The listing builds one solid part. Answer for the finished solid, in the listing's coordinates (mm). A direction names the side the tool comes from. Round coordinates to 2 decimals unless told otherwise and drop trailing zeros. Write each loop counter-clockwise with the first axis right and the second up, starting at its lowest first coordinate (ties: lowest second). Pieces come first, ordered by that corner, then holes. Notation, with made-up numbers: (25.25, -31) - (37.25, -31) arc R23 cw to (37.25, 2) - close; hole circle Ø6 at (19, 42.25). An arc over 180 degrees is marked (long way). Use a Markdown table: item, result. Add a question column.
1) Find the intervals of material crossed by probe 1 along X at (y, z) = (0.25, 1.25); probe 2 along Y at (x, z) = (0, 2.7) (3 decimals); probe 3 along X at (y, z) = (-0.25, 3.5), in increasing order. Write a range as from..to.
2) A tool of negligible diameter and unlimited length cuts with its end or side. For faces 4 (the flat face through (6, -6, -1.2)), 5 (the flat face through (57, 0, 7)), 6 (the cylindrical face through (-1.751, -7.883, 2.465)), from which of +Z, -Z, +X, -X, +Y, -Y can it reach the whole face along a straight path? Write none if from no direction.
3) A cutting plane is placed at B-B (x = 19). Give the vertices of the cut face in (y, z).
4) Each of these flat-tipped pins is pushed along its axis until it touches: P1, Ø5, axis at y = 8, z = 2, coming from the -X side; P2, Ø8, axis at x = 2.5, y = -2.5, coming from the -Z side; P3, Ø3, axis at y = -6.5, z = -0.5, coming from the +X side. Where does it stop, or does it pass through?
5) A cutting plane is placed at A-A (x = 94.5). Give the vertices of the cut face in (y, z).
6) Determine the mould class of faces 1 (the cylindrical face through (126, 0, 3)), 2 (the cylindrical face through (115.305, -1.532, -5.219)), 3 (the cylindrical face through (-7.995, 6.13, -1.521)) for opening direction X: +X half, -X half, draft (parallel to the pull), parting line (faces both ways), or undercut.
```python
from build123d import *

# Parameters (mm, degrees)
SKETCH_1_R          = 8.075
EXTRUDE_1_DEPTH     = 7
EXTRUDE_START       = -2
SKETCH_2_R          = 8.075
SKETCH_2_R_2        = 6.575
EXTRUDE_2_DEPTH     = 2
SKETCH_3_R          = 4
EXTRUDE_3_DEPTH     = 10
SKETCH_4_R          = 5
SKETCH_4_R_2        = 4
EXTRUDE_4_DEPTH     = 3
CHAMFER_1_SIZE      = 0.5
CUT_EXTRUDE_1_DEPTH = 7
CUT_EXTRUDE_2_DEPTH = 5
CUT_EXTRUDE_START   = -2
SKETCH_8_R          = 4
CUT_EXTRUDE_3_DEPTH = 2
FILLET_1_R          = 0.5
SKETCH_9_R          = 2.2
CUT_EXTRUDE_4_DEPTH = 10
EXTRUDE_START_2     = 3
SKETCH_10_R         = 10.075
SKETCH_10_R_2       = 8.075
EXTRUDE_5_DEPTH     = 3
EXTRUDE_6_DEPTH     = 2
EXTRUDE_START_3     = 5
EXTRUDE_7_DEPTH     = 5


with BuildPart() as part:
    # 草图1 → 凸台-拉伸1 (new body)
    with BuildSketch(Plane.XY):
        with BuildLine():
            ThreePointArc((0.37924895, 11.068504652), (-11.074999998, -0.000191538), (0.379631801, -11.068491528))
            Line((0.379631801, -11.068491528), (119, -7))
            ThreePointArc((119, -7), (125.998973572, -0.119870518), (119.239705882, 6.995894588))
            Line((119.239705882, 6.995894588), (0.37924895, 11.068504652))
        make_face()
        Circle(SKETCH_1_R, mode=Mode.SUBTRACT)
    extrude(amount=EXTRUDE_1_DEPTH)

    # 草图2 → 凸台-拉伸2 (add)
    with BuildSketch(Plane.XY.offset(7).offset(EXTRUDE_START)):
        Circle(SKETCH_2_R)
        Circle(SKETCH_2_R_2, mode=Mode.SUBTRACT)
    extrude(amount=EXTRUDE_2_DEPTH)

    # 草图3 → 凸台-拉伸3 (add)
    with BuildSketch(Plane(origin=(0, 0, 0), x_dir=(-1, 0, 0), z_dir=(0, 0, -1))):
        with Locations((-119, 0)):
            Circle(SKETCH_3_R)
    extrude(amount=EXTRUDE_3_DEPTH)

    # 草图4 → 凸台-拉伸4 (add)
    with BuildSketch(Plane(origin=(0, 0, 0), x_dir=(-1, 0, 0), z_dir=(0, 0, -1))):
        with Locations(Location((-119, 0, 0), (0, 0, 180))):
            Circle(SKETCH_4_R)
        with Locations((-119, 0)):
            Circle(SKETCH_4_R_2, mode=Mode.SUBTRACT)
    extrude(amount=EXTRUDE_4_DEPTH)

    # 倒角1
    chamfer_1_edges = [part.edges().sort_by_distance(p)[0] for p in [
        (-6.575, 0, 5),
        (-6.575, 0, 7),
        (123, 0, -10),
        (114, 0, -3),
    ]]
    chamfer(chamfer_1_edges, length=CHAMFER_1_SIZE)

    # 草图5 → 切除-拉伸1 (cut)
    with BuildSketch(Plane(origin=(0, 0, 0), x_dir=(-1, 0, 0), z_dir=(0, 0, -1))):
        with BuildLine():
            ThreePointArc((-12.757234161, -4.640431182), (-13.574999998, 0.000234775), (-12.757073645, 4.640872443))
            Line((-12.757073645, 4.640872443), (-109.090204802, 1.340134001))
            ThreePointArc((-109.090204802, 1.340134001), (-109.022576686, 0.671583213), (-109, 0))
            ThreePointArc((-109, 0), (-109.022449652, -0.669693251), (-109.08969781, -1.336379625))
            Line((-109.08969781, -1.336379625), (-12.757234161, -4.640431182))
        make_face()
    extrude(amount=-CUT_EXTRUDE_1_DEPTH, mode=Mode.SUBTRACT)

    # 草图6 → 切除-拉伸2 (cut)
    with BuildSketch(Plane(origin=(0, 0, 0), x_dir=(-1, 0, 0), z_dir=(0, 0, -1))):
        Polygon((-109.08969781, -1.336379625), (-12.757234161, -4.640431182), (-12.860068961, -7.638668165), (-109.192532609, -4.334616608), align=None)
        Polygon((-12.757073645, 4.640872443), (-109.090204802, 1.340134001), (-109.192935895, 4.338374538), (-12.859804737, 7.63911298), align=None)
    extrude(amount=-CUT_EXTRUDE_2_DEPTH, mode=Mode.SUBTRACT)

    # 草图8 → 切除-拉伸3 (cut)
    with BuildSketch(Plane(origin=(0, 0, -10), x_dir=(-1, 0, 0), z_dir=(0, 0, -1)).offset(CUT_EXTRUDE_START)):
        with Locations((-119, 0)):
            Circle(SKETCH_8_R)
    extrude(amount=CUT_EXTRUDE_3_DEPTH, mode=Mode.SUBTRACT)

    # 圆角1
    fillet_1_edges = [part.edges().sort_by_distance(p)[0] for p in [
        (123, 0, -8),
    ]]
    fillet(fillet_1_edges, radius=FILLET_1_R)

    # 草图9 → 切除-拉伸4 (cut)
    with BuildSketch(Plane(origin=(0, 0, -8), x_dir=(-1, 0, 0), z_dir=(0, 0, -1))):
        with Locations((-119, 0)):
            Circle(SKETCH_9_R)
    extrude(amount=-CUT_EXTRUDE_4_DEPTH, mode=Mode.SUBTRACT)

    # 草图10 → 凸台-拉伸5 (add)
    with BuildSketch(Plane(origin=(0, 0, 0), x_dir=(-1, 0, 0), z_dir=(0, 0, -1)).offset(EXTRUDE_START_2)):
        with Locations(Location((0, 0, 0), (0, 0, 180))):
            Circle(SKETCH_10_R)
        Circle(SKETCH_10_R_2, mode=Mode.SUBTRACT)
    extrude(amount=-EXTRUDE_5_DEPTH)

    # 切除-旋转2: read off the stored shape, not the designer's step
    # 切除-旋转2: loft between two sections, ruled curve by curve
    cut_revolve_2_from = [
        Edge.make_three_point_arc((8.65, 0, -1.2), (0, 8.65, -1.2), (-8.65, 0, -1.2)),
        Edge.make_three_point_arc((-8.65, 0, -1.2), (0, -8.65, -1.2), (8.65, 0, -1.2)),
    ]
    cut_revolve_2_to = [
        Edge.make_three_point_arc((8.65, 0, 0), (0, 8.65, 0), (-8.65, 0, 0)),
        Edge.make_three_point_arc((-8.65, 0, 0), (0, -8.65, 0), (8.65, 0, 0)),
    ]
    cut_revolve_2 = Solid(Shell([*[Face.make_surface_from_curves(cut_revolve_2_from[k], cut_revolve_2_to[k]) for k in range(2)], Face(Wire(cut_revolve_2_from)), Face(Wire(cut_revolve_2_to))]))
    add(cut_revolve_2, mode=Mode.SUBTRACT)

    # 草图12 → 凸台-拉伸6 (add)
    with BuildSketch(Plane.XY.offset(7).offset(EXTRUDE_START)):
        with BuildLine():
            Line((109.08969781, -1.336379625), (12.757234161, -4.640431182))
            ThreePointArc((12.757234161, -4.640431182), (13.574999998, 0.000234775), (12.757073645, 4.640872443))
            Line((12.757073645, 4.640872443), (109.090204802, 1.340134001))
            ThreePointArc((109.090204802, 1.340134001), (109.000000179, 0.001894226), (109.08969781, -1.336379625))
        make_face()
    extrude(amount=EXTRUDE_6_DEPTH)

    # 草图13 → 凸台-拉伸7 (add)
    with BuildSketch(Plane(origin=(0, 0, 5), x_dir=(-1, 0, 0), z_dir=(0, 0, -1)).offset(EXTRUDE_START_3)):
        with BuildLine():
            Line((-109.08969781, -1.336379625), (-109.192532609, -4.334616608))
            Line((-109.192532609, -4.334616608), (-12.860068961, -7.638668165))
            Line((-12.860068961, -7.638668165), (-12.757234161, -4.640431182))
            ThreePointArc((-12.757234161, -4.640431182), (-13.574999998, 0.000234775), (-12.757073645, 4.640872443))
            Line((-12.757073645, 4.640872443), (-12.859804737, 7.63911298))
            Line((-12.859804737, 7.63911298), (-109.192935895, 4.338374538))
            Line((-109.192935895, 4.338374538), (-109.090204802, 1.340134001))
            ThreePointArc((-109.090204802, 1.340134001), (-109.000000179, 0.001894226), (-109.08969781, -1.336379625))
        make_face()
    extrude(amount=-EXTRUDE_7_DEPTH)


solid = part.part
```
Entries:
| question | item | result |
|---|---|---|
| 1 | probe 1 | x = -11.07..-8.07, 8.07..116.81, 121.19..126 |
| 1 | probe 2 | y = -11.075..-8.075, 8.075..11.075 |
| 1 | probe 3 | x = -11.07..-8.07, 8.07..126 |
| 2 | face 4 | none |
| 2 | face 5 | +Z, +X, -X, +Y, -Y |
| 2 | face 6 | -Z |
| 3 | outline | (-10.43, 0) - (10.43, 0) - (10.43, 7) - (-10.43, 7) - close |
| 4 | P1 | stops at x = -9.61 |
| 4 | P2 | stops at z = 5 |
| 4 | P3 | stops at x = 123.81 |
| 5 | outline | (-7.84, 0) - (7.84, 0) - (7.84, 7) - (-7.84, 7) - close |
| 6 | face 1 | +X half |
| 6 | face 2 | parting line |
| 6 | face 3 | undercut |
